Autodesk Fusion 360 part; units mm, degrees
sketch "Skizze1" plane through (0, 0, 0) normal (0, 1, 0) x (1, 0, 0)
  line L0 (0, 0) -> (7, 0)
  line L1 (7, 0) -> (7, -65)
  line L2 (7, -65) -> (0, -65)
  line L3 (0, -65) -> (0, 0)
  dimension "d1" = 7
  dimension "d2" = 65
extrude "Extrusion1" add sketch "Skizze1" along normal blind 1.5
sketch "Skizze2" plane through (0, 1.5, 0) normal (0, 1, 0) x (-1, 0, 0)
  line L0 (0, 65) -> (-7, 65)
  line L1 (-7, 65) -> (-7, 0)
  line L2 (-7, 0) -> (0, 0)
  line L3 (0, 0) -> (0, 65)
  line L4 (-1.5, 65) -> (-1.5, 0)
  dimension "d5" = 1.5
extrude "Extrusion2" add sketch "Skizze2" along normal blind 21 contours L0 L2 L3 L4
fillet "Abrundung1" radius 4 4 edges at (0.75, 22.5, 65) (7, 0.75, 65) (0.75, 22.5, 0) (7, 0.75, 0)
sketch "Skizze3" plane through (1.5, 0, 0) normal (1, 0, 0) x (0, 1, 0)
  arc A0 (18.5, 0) -> (22.5, 4) centre (18.5, 4) ccw
  line L0 (22.5, 4) -> (22.5, 61)
  arc A1 (22.5, 61) -> (18.5, 65) centre (18.5, 61) ccw
  line L1 (18.5, 65) -> (1.5, 65)
  line L2 (1.5, 65) -> (1.5, 0)
  line L3 (1.5, 0) -> (18.5, 0)
  line L4 (12, 65) -> (12, 0)
  circle A2 centre (12, 50) radius 2.5
  circle A3 centre (12, 15) radius 2.5
  dimension "d10" = 12
  dimension "d11" = 5
  dimension "d12" = 5
  dimension "d13" = 15
  dimension "d14" = 15
extrude "Extrusion3" cut sketch "Skizze3" against normal blind 2 contours L4 A3 | L4 A3 | L4 A2 | L4 A2
chamfer "Fase1" distance 0.5 angle 45 2 edges at (0, 9.6692, 49.096) (0, 9.6692, 14.096)
fillet "Abrundung4" radius 0.4 1 edges at (1.5, 1.5, 32.5)
fillet "Abrundung6" radius 1 1 edges at (0, 0, 32.5)
fillet "Abrundung7" radius 0.3 26 edges at (1.5, 22.5, 32.5) (1.5, 21.3284, 1.1716) (1.5, 10.2, 0) (1.6172, 1.6172, 0) (2.45, 1.5, 0) (5.8284, 1.5, 1.1716) (7, 1.5, 32.5) (5.8284, 1.5, 63.8284) (2.45, 1.5, 65) (1.6172, 1.6172, 65) (1.5, 10.2, 65) (1.5, 21.3284, 63.8284) (0, 21.3284, 63.8284) (0, 9.75, 65) (0.2929, 0.2929, 65) (2, 0, 65) (5.8284, 0, 63.8284) (7, 0, 32.5) (5.8284, 0, 1.1716) (2, 0, 0) (0.2929, 0.2929, 0) (0, 9.75, 0) (0, 21.3284, 1.1716) (0, 22.5, 32.5) (1.5, 9.6692, 50.904) (1.5, 9.6692, 15.904)
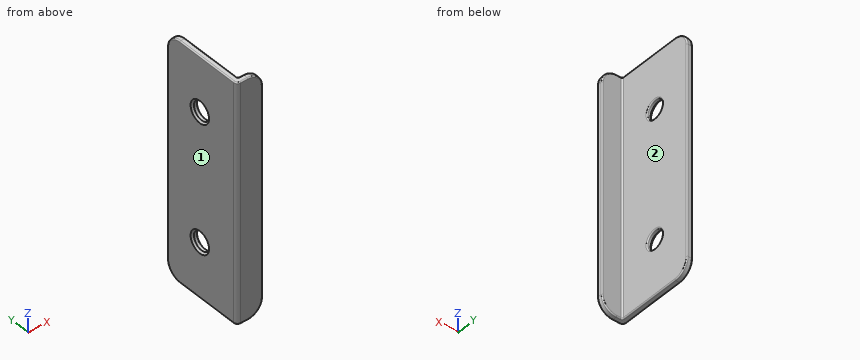
Check sheet for the modelled part. Datum: model origin and axes. Units: mm. Face numbers are marked on the shaded views. A direction names the side the tool comes from. Round coordinates to 2 decimals unless told otherwise and drop trailing zeros. Order: outer loops, then holes, each group sorted by start corner. A loop starts at its lowest first (then second) coordinate and runs counter-clockwise, first axis right, second up. Notation, with made-up numbers: M 37,37.25 L 65,37.25 A27 ccw 65,73.25 Z; hole C 56.25,71.5 d4. An arc over 180 degrees is marked long. Answer in a Markdown table with one row per item.
(1) Material ranges on line 1 along Z through (x, y) = (1, 12); line 2 along Y through (x, z) = (0.85, 15); line 3 along Y through (x, z) = (2.5, 28), recorded low to high. Write a range as from..to.
Findings:
| item | result |
|---|---|
| line 1 | z = 0..12.5, 17.5..47.5, 52.5..65 |
| line 2 | y = 0.01..9.5, 14.5..22.5 |
| line 3 | y = 0..1.5 |
(2) Section check A-A on y = 12. Record the boundary of the cut face in (x, z), plus the area to 3 significant figures.
Findings:
| item | result |
|---|---|
| outline | M 0,0.3 A0.3 ccw 0.3,0 L 1.2,0 A0.3 ccw 1.5,0.3 L 1.5,12.2 A0.3 ccw 1.2,12.5 L 0.5,12.5 L 0,12 Z; M 0,18 L 0.5,17.5 L 1.2,17.5 A0.3 ccw 1.5,17.8 L 1.5,47.2 A0.3 ccw 1.2,47.5 L 0.5,47.5 L 0,47 Z; M 0,53 L 0.5,52.5 L 1.2,52.5 A0.3 ccw 1.5,52.8 L 1.5,64.7 A0.3 ccw 1.2,65 L 0.3,65 A0.3 ccw 0,64.7 Z |
| area | 81.8 mm^2 |
(3) Set-up check for the marked faces 1 and 2: record each of +Z, -Z, +X, -X, +Y, -Y from which the full face is reachable in a straight line by a thin tool's end or side.
Findings:
| item | result |
|---|---|
| face 1 | +Z, -Z, -X, +Y, -Y |
| face 2 | +Z, -Z, +X, +Y |
(4) Section check B-B on z = 15. Record the boundary of the cut face in (x, y).
Findings:
| item | result |
|---|---|
| outline | M 0,1 A1 ccw 1,0 L 6.7,0 A0.3 ccw 7,0.3 L 7,1.2 A0.3 ccw 6.7,1.5 L 1.9,1.5 A0.4 cw 1.5,1.9 L 1.5,9.2 A0.3 ccw 1.2,9.5 L 0.5,9.5 L 0,9 Z; M 0,15 L 0.5,14.5 L 1.2,14.5 A0.3 ccw 1.5,14.8 L 1.5,22.2 A0.3 ccw 1.2,22.5 L 0.3,22.5 A0.3 ccw 0,22.2 Z |
(5) Section check C-C on z = 54. Record the boundary of the cut face in (x, y).
Findings:
| item | result |
|---|---|
| outline | M 0,1 A1 ccw 1,0 L 6.7,0 A0.3 ccw 7,0.3 L 7,1.2 A0.3 ccw 6.7,1.5 L 1.9,1.5 A0.4 cw 1.5,1.9 L 1.5,22.2 A0.3 ccw 1.2,22.5 L 0.3,22.5 A0.3 ccw 0,22.2 Z |
(6) Gauge pin test, flat ends, axial feed: pin 1 (4.5 mm diameter, centred on y = 12, z = 50, fed in from +X); pin 2 (4 mm diameter, centred on x = 5, z = 35.5, fed in from +Y); pin 3 (8 mm diameter, centred on y = 19, z = 42.5, fed in from +X). Record the tip position at first contact, or that the pin passes through.
Findings:
| item | result |
|---|---|
| pin 1 | passes through |
| pin 2 | stops at y = 1.5 |
| pin 3 | stops at x = 1.5 |
